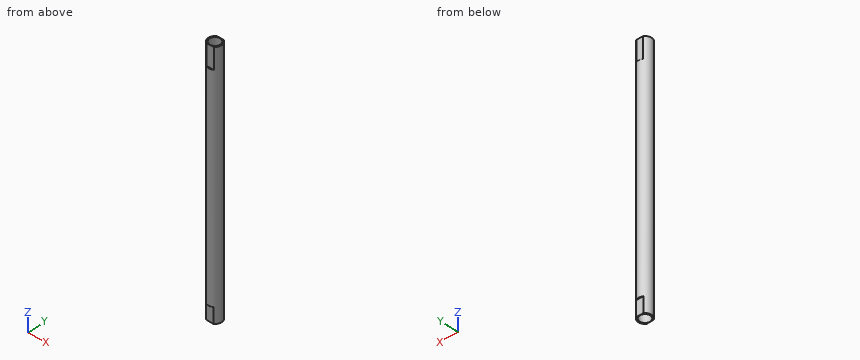
from build123d import *

# Parameters (mm, degrees)
SKETCH2_R           = 13.383565171
SKETCH2_R_2         = 10.769869961
BOSS_EXTRUDE1_DEPTH = 508
CUT_EXTRUDE1_START  = -41.91
CUT_EXTRUDE1_DEPTH  = 41.91
CUT_EXTRUDE2_DEPTH  = 30.988


with BuildPart() as part:
    # Sketch2 → Boss-Extrude1 (new body)
    with BuildSketch(Plane.XY):
        Circle(SKETCH2_R)
        Circle(SKETCH2_R_2, mode=Mode.SUBTRACT)
    extrude(amount=BOSS_EXTRUDE1_DEPTH)

    # Sketch3 → Cut-Extrude1 (cut)
    with BuildSketch(Plane.XY.offset(508).offset(CUT_EXTRUDE1_START)):
        with BuildLine():
            ThreePointArc((6.70741417, 11.581468466), (0, 13.383565171), (-6.70741417, 11.581468466))
            Line((-6.70741417, 11.581468466), (6.70741417, 11.581468466))
        make_face()
        with BuildLine():
            Line((7.648089194, -10.983011807), (-6.70741417, -11.581468466))
            ThreePointArc((-6.70741417, -11.581468466), (0.557454006, -13.371950557), (7.648089194, -10.983011807))
        make_face()
    extrude(amount=CUT_EXTRUDE1_DEPTH, mode=Mode.SUBTRACT)

    # Sketch4 → Cut-Extrude2 (cut)
    with BuildSketch(Plane(origin=(0, 0, 0), x_dir=(-1, 0, 0), z_dir=(0, 0, -1))):
        with BuildLine():
            ThreePointArc((7.196946438, 11.28378388), (0, 13.383565171), (-7.196946438, 11.28378388))
            Line((-7.196946438, 11.28378388), (7.196946438, 11.28378388))
        make_face()
        with BuildLine():
            Line((7.820080378, -10.861222747), (-7.196946438, -11.28378388))
            ThreePointArc((-7.196946438, -11.28378388), (0.376448475, -13.378269814), (7.820080378, -10.861222747))
        make_face()
    extrude(amount=-CUT_EXTRUDE2_DEPTH, mode=Mode.SUBTRACT)


solid = part.part
For this review, take the finished solid that the model builds, in its own axes (mm). Coordinates: 2 decimals unless noted, no trailing zeros. Loops run counter-clockwise (first coordinate to the right, second up) from the corner with the lowest first, then second, coordinate; pieces in that order, holes last. Notation, with made-up numbers: (77.5, -10) - (86.5, -10) arc R14 cw to (86.5, 14) - close; hole circle Ø8 at (-32.5, 40). An arc over 180 degrees is marked (long way). Use a Markdown table: item, result. Add a question column.
Item 1: We need section C-C (z = 277.5). Give the boundary of the cut face in (x, y), and give its area (3 significant figures).
Item 2: We need section A-A (y = 0). Give the boundary of the cut face in (x, z), and give its area (3 significant figures).
Item 3: For line 1 (Y direction, x = 0, z = 324); line 2 (X direction, y = -8, z = 191); line 3 (Y direction, x = 6.5, z = 378), list the stretches that pass through material, from the lowest coordinate up.
Item 4: Insertion check: pin 1 Ø0.8 at (x, y) = (-0.5, -12.5) entering from -Z; pin 2 Ø11.5 at (x, z) = (-1.5, 12) entering from +Y; pin 3 Ø6.5 at (x, z) = (0, 483.5) entering from +Y; pin 4 Ø1.9 at (x, y) = (4, -12) entering from +Z. Each pin has a flat end and moves straight along its axis. Give the tip position at first contact, or say it passes through.
Item 5: We need section B-B (x = 0). Give the boundary of the cut face in (y, z), and give its area (3 significant figures).
Results list:
| question | item | result |
|---|---|---|
| 1 | outline | circle Ø26.77 at (0, 0); hole circle Ø21.54 at (0, 0) |
| 1 | area | 198 mm^2 |
| 2 | outline | (-13.38, 0) - (-10.77, 0) - (-10.77, 508) - (-13.38, 508) - close; (10.77, 0) - (13.38, 0) - (13.38, 508) - (10.77, 508) - close |
| 2 | area | 2,660 mm^2 |
| 3 | line 1 | y = -13.38 to -10.77, 10.77 to 13.38 |
| 3 | line 2 | x = -10.73 to -7.21, 7.21 to 10.73 |
| 3 | line 3 | y = -11.7 to -8.59, 8.59 to 11.7 |
| 4 | pin 1 | stops at z = 30.99 |
| 4 | pin 2 | stops at y = 11.28 |
| 4 | pin 3 | stops at y = 11.58 |
| 4 | pin 4 | stops at z = 508 |
| 5 | outline | (-13.38, 30.99) - (-11.08, 30.99) - (-11.08, 0) - (-10.77, 0) - (-10.77, 508) - (-11.3, 508) - (-11.3, 466.09) - (-13.38, 466.09) - close; (10.77, 0) - (11.28, 0) - (11.28, 30.99) - (13.38, 30.99) - (13.38, 466.09) - (11.58, 466.09) - (11.58, 508) - (10.77, 508) - close |
| 5 | area | 2,360 mm^2 |
